Geometry check sheet. Reference: drawing and pictorial views, mm from the part's lowest x, y, z. Coordinates: 2 decimals unless noted, no trailing zeros. Write each loop counter-clockwise with the first axis right and the second up, starting at its lowest first coordinate (ties: lowest second). Pieces come first, ordered by that corner, then holes. Notation, with made-up numbers: (-5, -36.75) - (27, -36.75) arc R24 cw to (27, -21.75) - close; hole circle Ø2 at (43.25, -3). An arc over 180 degrees is marked (long way). Use one line per item in the form item = value. Start each with the question number.
(1) Sectioned sample at C-C (x = 35). Record the cut outline in (y, z), and give its area (4 significant figures).
(2) Material ranges on line 1 (Y direction, x = 19, z = 4.75); line 2 (Y direction, x = 35, z = 1.5); line 3 (Z direction, x = 10, y = 12), recorded low to high. Write a range as [from, to].
(3) Sectioned sample at A-A (z = 2). Record the cut outline in (x, y).
(4) Mould release check, pull along Y, two halves, no side actions. Record for the marked faces 1, 2 and 3: released by +Y, released by -Y, zero draft, split by the parting line, or undercut.
(5) Sectioned sample at B-B (y = 23). Record the cut outline in (x, z), and give its area (3 significant figures).
(6) Gauge pin test, flat ends, axial feed: pin 1 Ø11.5 at (x, y) = (11.5, 51) entering from -Z; pin 2 Ø4 at (y, z) = (14, 3) entering from -X; pin 3 Ø2 at (x, z) = (35, 4) entering from +Y. Record the tip position at first contact, or that the pin passes through.
(7) Sectioned sample at D-D (x = 19). Record the cut outline in (y, z), and give its area (4 significant figures).
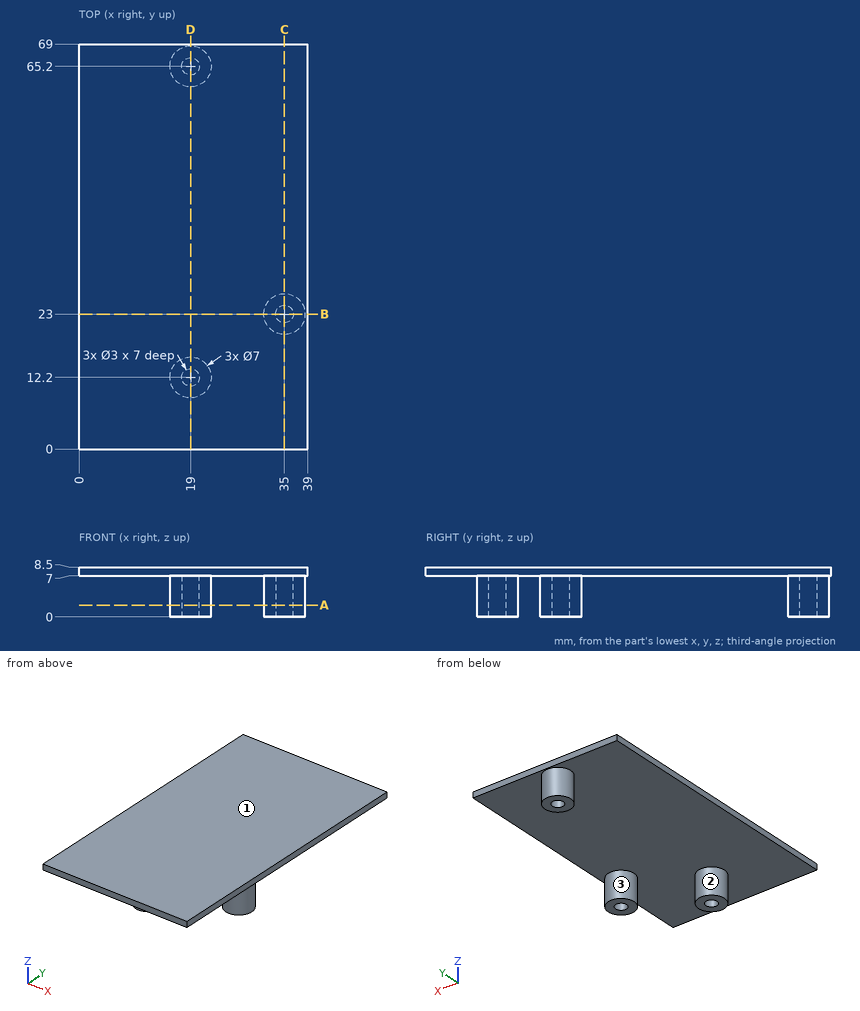
Answers below:
q1.outline = (0, 7) - (19.5, 7) - (19.5, 0) - (21.5, 0) - (21.5, 7) - (24.5, 7) - (24.5, 0) - (26.5, 0) - (26.5, 7) - (69, 7) - (69, 8.5) - (0, 8.5) - close
q1.area = 131.5 mm2
q2.line_1 = [8.7, 10.7], [13.7, 15.7], [61.7, 63.7], [66.7, 68.7]
q2.line_2 = [19.5, 21.5], [24.5, 26.5]
q2.line_3 = [7, 8.5]
q3.outline = circle Ø7 at (19, 12.2); circle Ø7 at (19, 65.2); circle Ø7 at (35, 23); hole circle Ø3 at (19, 12.2); hole circle Ø3 at (19, 65.2); hole circle Ø3 at (35, 23)
q4.face_1 = zero draft
q4.face_2 = undercut
q4.face_3 = split by the parting line
q5.outline = (0, 7) - (31.5, 7) - (31.5, 0) - (33.5, 0) - (33.5, 7) - (36.5, 7) - (36.5, 0) - (38.5, 0) - (38.5, 7) - (39, 7) - (39, 8.5) - (0, 8.5) - close
q5.area = 86.5 mm2
q6.pin_1 = 7
q6.pin_2 = 15.5
q6.pin_3 = 26.5
q7.outline = (0, 7) - (8.7, 7) - (8.7, 0) - (10.7, 0) - (10.7, 7) - (13.7, 7) - (13.7, 0) - (15.7, 0) - (15.7, 7) - (61.7, 7) - (61.7, 0) - (63.7, 0) - (63.7, 7) - (66.7, 7) - (66.7, 0) - (68.7, 0) - (68.7, 7) - (69, 7) - (69, 8.5) - (0, 8.5) - close
q7.area = 159.5 mm2
